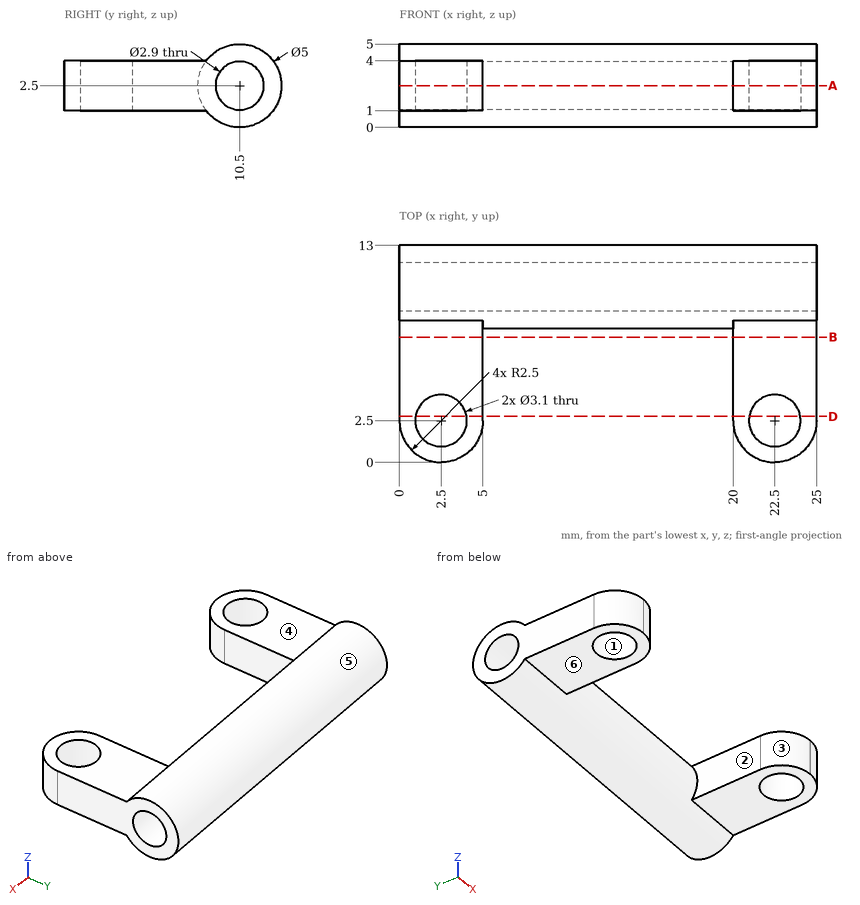
Design review of the part shown in the three views and the two pictorial views. Dimensions are in mm from the part's minimum x, y and z. A direction names the side the tool comes from. Round coordinates to 2 decimals unless told otherwise and drop trailing zeros. Write each loop counter-clockwise with the first axis right and the second up, starting at its lowest first coordinate (ties: lowest second). Pieces come first, ordered by that corner, then holes. Notation, with made-up numbers: (81, -29.5) - (86, -29.5) arc R36 ccw to (86, 6.5) - close; hole circle Ø9 at (23.5, 74). An arc over 180 degrees is marked (long way). Write item = value, one per line. Start each with the question number.
1. Consider section A-A on z = 2.5. Give the number of separate pieces and of enclosed holes in the cut face, plus the area to 3 significant figures.
2. Draft analysis for pull direction Y (two halves, no side actions). For the marked faces 1, 2 and 3, state which applies: released by +Y, released by -Y, zero draft, split by the parting line, or undercut.
3. For pin 1 Ø2.5 at (x, y) = (1.5, 3) entering from +Z; pin 2 Ø1.5 at (x, y) = (21, 4.5) entering from -Z, all flat-tipped, find the tip position at first contact; note any pin that passes through.
4. Consider section D-D on y = 2.75. State the section outline as (x, z) points.
5. For the marked faces 4, 5 and 6, list the 3-axis set-ups (+Z, -Z, +X, -X, +Y, -Y) from which the entire face can be reached by the end or side of a thin tool; tool diameter is ignored.
6. Consider section B-B on y = 7.5. State the section outline as (x, z) points.
7. Wall thickness on L1, parallel to Y at x = 2.5, z = 2.45; L2, parallel to X at y = 6, z = 2; L3, parallel to X at y = 3, z = 3.1: over which ranges is each line inside the solid? List them lowest first.
Evaluation:
q1.separate_pieces = 2
q1.enclosed_holes = 2
q1.area = 112 mm2
q2.face_1 = undercut
q2.face_2 = zero draft
q2.face_3 = released by -Y
q3.pin_1 = 4
q3.pin_2 = 1
q4.outline = (0, 1) - (0.97, 1) - (0.97, 4) - (0, 4) - close; (4.03, 1) - (5, 1) - (5, 4) - (4.03, 4) - close; (20, 1) - (20.97, 1) - (20.97, 4) - (20, 4) - close; (24.03, 1) - (25, 1) - (25, 4) - (24.03, 4) - close
q5.face_4 = +Z, +X, -X, -Y
q5.face_5 = none
q5.face_6 = -Z, +X, -X, -Y
q6.outline = (0, 1) - (5, 1) - (5, 4) - (0, 4) - close; (20, 1) - (25, 1) - (25, 4) - (20, 4) - close
q7.L1 = 0 to 0.95, 4.05 to 9.05, 11.95 to 13
q7.L2 = 0 to 5, 20 to 25
q7.L3 = 0 to 1.03, 3.97 to 5, 20 to 21.03, 23.97 to 25
